Check sheet for the modelled part. Datum: model origin and axes. Units: mm. Round coordinates to 2 decimals unless told otherwise and drop trailing zeros. Write each loop counter-clockwise with the first axis right and the second up, starting at its lowest first coordinate (ties: lowest second). Pieces come first, ordered by that corner, then holes. Notation, with made-up numbers: M 86.25,31.25 L 130.25,31.25 A7 ccw 130.25,35.25 Z; hole C 85.25,82 d4. An arc over 180 degrees is marked long. Answer in a Markdown table with one row per item.
Autodesk Inventor part; units mm, degrees
ref_plane "YZ Plane" through (0, 0, 0) normal (1, 0, 0) x (0, 1, 0)
ref_plane "XZ Plane" through (0, 0, 0) normal (0, 1, 0) x (-1, 0, 0)
ref_plane "XY Plane" through (0, 0, 0) normal (0, 0, 1) x (1, 0, 0)
sketch "Sketch1" plane through (0, 0, 0) normal (0, 1, 0) x (-1, 0, 0)
  line L0 (42.2226, 53.0438) -> (-12.2774, 53.0438)
  line L1 (-12.2774, 53.0438) -> (-12.2774, -29.9562)
  line L2 (-12.2774, -29.9562) -> (42.2226, -29.9562)
  line L3 (42.2226, -29.9562) -> (42.2226, 53.0438)
  point P0 (0, 0)
  dimension "d0" = 54.5
  dimension "d1" = 83
extrude "Extrusion1" add sketch "Sketch1" along normal blind 2.35
sketch "Sketch2" plane through (0, 2.35, 0) normal (0, 1, 0) x (1, 0, 0)
  line L0 (-39.8226, -46.2538) -> (9.1374, -46.2538)
  line L1 (9.1374, -46.2538) -> (9.1374, 27.1862)
  line L2 (9.1374, 27.1862) -> (-39.8226, 27.1862)
  line L3 (-39.8226, 27.1862) -> (-39.8226, -46.2538)
  line L4 (12.2774, -53.0438) -> (12.2774, 29.9562)
  line L5 (12.2774, 29.9562) -> (-42.2226, 29.9562)
  line L6 (-42.2226, 29.9562) -> (-42.2226, -53.0438)
  line L7 (-42.2226, -53.0438) -> (12.2774, -53.0438)
  point P0 (0, 0)
  dimension "d4" = 48.96
  dimension "d5" = 73.44
  dimension "d6" = 2.77
  dimension "d7" = 2.4
extrude "Extrusion2" add sketch "Sketch2" along normal blind 0.1 contours L3 L2 L1 L0
sketch "Sketch3" plane through (0, 0, 0) normal (0, -1, 0) x (1, 0, 0)
  line L0 (12.2774, 53.0438) -> (12.2774, -29.9562)
  line L1 (-42.2226, 53.0438) -> (12.2774, 53.0438)
  line L2 (-42.2226, -29.9562) -> (-42.2226, 53.0438)
  line L3 (12.2774, -29.9562) -> (-42.2226, -29.9562)
  line L4 (-42.2226, 53.0438) -> (12.2774, 53.0438)
  line L5 (-32.3226, 53.0438) -> (-32.3226, 31.8438)
  line L6 (-32.3226, 31.8438) -> (-11.8226, 31.8438)
  line L7 (-11.8226, 31.8438) -> (-11.8226, 43.0438)
  line L8 (-11.8226, 43.0438) -> (8.2974, 43.0438)
  line L9 (8.2974, 43.0438) -> (8.2974, 53.0438)
  point P0 (0, 0)
  dimension "d11" = 9.9
  dimension "d12" = 21.2
  dimension "d13" = 3.98
  dimension "d14" = 20.5
  dimension "d15" = 10
extrude "Extrusion3" add sketch "Sketch3" along normal blind 4.3 contours L9 L8 L7 L6 L5 L1
fillet "Fillet2" radius 3 1 edges at (-12.0126, -4.3, 53.0438)
sketch "Sketch4" plane through (-11.8226, 0, 31.8438) normal (0, 0, -1) x (-1, 0, 0)
  line L0 (0, 0) -> (20.5, 0)
  line L1 (0, 0) -> (0, -4.3)
  line L2 (20.5, -4.3) -> (0, -4.3)
  line L3 (20.5, 0) -> (20.5, -4.3)
  line L4 (0, -2.3) -> (20.5, -2.3)
  line L5 (20.5, -1.3) -> (20.5, -4.3)
  point P0 (-11.8226, 0)
  point P1 (0, -2.3)
  dimension "d19" = 2
extrude "Extrusion4" cut sketch "Sketch4" against normal blind 3.5 contours L4 L3 L2 L1
properties part number "Display"
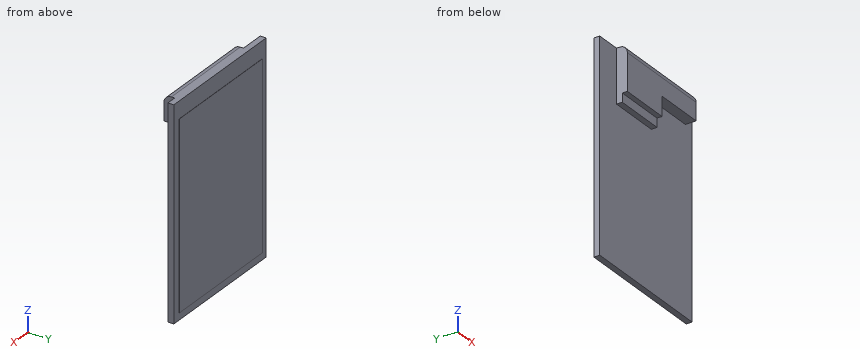
1. Scan lines: L1, parallel to Y at x = -7.5, z = -7; L2, parallel to Z at x = -7.5, y = -0.75; L3, parallel to Y at x = 6.5, z = 49. Record each from-to range of solid material in increasing order.
Found:
| item | result |
|---|---|
| L1 | y = 0 to 2.45 |
| L2 | z = 43.04 to 53.04 |
| L3 | y = -4.3 to 2.35 |
2. Section check A-A, the plane x = -19.5. Record the cut outline in (y, z).
Found:
| item | result |
|---|---|
| outline | M -4.3,35.34 L -2.3,35.34 L -2.3,31.84 L 0,31.84 L 0,-29.96 L 2.35,-29.96 L 2.35,-27.19 L 2.45,-27.19 L 2.45,46.25 L 2.35,46.25 L 2.35,53.04 L -1.3,53.04 A3 ccw -4.3,50.04 Z |
3. Go/stop test with flat-tipped pins: pin 1 (3.5 mm diameter, centred on y = -2, z = 50, fed in from +X); pin 2 (2 mm diameter, centred on x = -24, y = -3.5, fed in from -Z); pin 3 (2 mm diameter, centred on y = -2, z = 39.5, fed in from +X). Record where each tip stops, or that it passes through.
Found:
| item | result |
|---|---|
| pin 1 | stops at x = 8.3 |
| pin 2 | stops at z = 35.34 |
| pin 3 | stops at x = -11.82 |
4. Section check B-B, the plane z = 42. Record the cut outline in (x, y).
Found:
| item | result |
|---|---|
| outline | M -42.22,0 L -32.32,0 L -32.32,-4.3 L -11.82,-4.3 L -11.82,0 L 12.28,0 L 12.28,2.35 L 9.14,2.35 L 9.14,2.45 L -39.82,2.45 L -39.82,2.35 L -42.22,2.35 Z |
5. Section check C-C, the plane x = -6. Record the cut outline in (y, z), and give its area (3 significant figures).
Found:
| item | result |
|---|---|
| outline | M -4.3,43.04 L 0,43.04 L 0,-29.96 L 2.35,-29.96 L 2.35,-27.19 L 2.45,-27.19 L 2.45,46.25 L 2.35,46.25 L 2.35,53.04 L -1.3,53.04 A3 ccw -4.3,50.04 Z |
| area | 243 mm2 |
6. Section check D-D, the plane z = 2. Record the cut outline in (x, y), and give its area (3 significant figures).
Found:
| item | result |
|---|---|
| outline | M -42.22,0 L 12.28,0 L 12.28,2.35 L 9.14,2.35 L 9.14,2.45 L -39.82,2.45 L -39.82,2.35 L -42.22,2.35 Z |
| area | 133 mm2 |
